Could you check a few things on this model? Use its own coordinates, in mm. A direction names the side the tool comes from. Round coordinates to 2 decimals unless told otherwise and drop trailing zeros. Write each loop counter-clockwise with the first axis right and the second up, starting at its lowest first coordinate (ties: lowest second). Pieces come first, ordered by that corner, then holes. Notation, with made-up numbers: (-12, 87.25) -> (14, 87.25) arc R16 ccw to (14, 94.25) -> close; hole circle Ø4 at (0.5, -15). An arc over 180 degrees is marked (long way). Answer in a Markdown table with one row per item.
from build123d import *

# Parameters (mm, degrees)
CUT_EXTRUDE1_START = -0.1
SKETCH2_R          = 7.95
SKETCH2_R_2        = 6.75
CUT_EXTRUDE1_DEPTH = 0.1


with BuildPart() as part:
    # Sketch1 → Revolve1 (revolve)
    with BuildSketch(Plane(origin=(0, 0, 0), x_dir=(0, 0, -1), z_dir=(1, 0, 0))):
        Polygon((0, 20), (9, 20), (9, 15.5), (8, 15.5), (8, 5), (6.75, 5), (6.75, 0), (0, 0), align=None)
    revolve(axis=Axis((0, 0, 0), (0, 1, 0)))

    # Sketch2 → Cut-Extrude1 (cut)
    with BuildSketch(Plane(origin=(0, 20, 0), x_dir=(1, 0, 0), z_dir=(0, 1, 0)).offset(CUT_EXTRUDE1_START)):
        with Locations(Location((0, 0, 0), (0, 0, 270))):
            Circle(SKETCH2_R)
        with Locations(Location((0, 0, 0), (0, 0, 90))):
            Circle(SKETCH2_R_2, mode=Mode.SUBTRACT)
    extrude(amount=CUT_EXTRUDE1_DEPTH, mode=Mode.SUBTRACT)


solid = part.part
1) Imagine slicing it at A-A, the plane x = 0. Please give me the cut outline in (y, z), plus the area to 3 significant figures.
Findings:
| item | result |
|---|---|
| outline | (0, -6.75) -> (5, -6.75) -> (5, -8) -> (15.5, -8) -> (15.5, -9) -> (20, -9) -> (20, -7.95) -> (19.9, -7.95) -> (19.9, -6.75) -> (20, -6.75) -> (20, 6.75) -> (19.9, 6.75) -> (19.9, 7.95) -> (20, 7.95) -> (20, 9) -> (15.5, 9) -> (15.5, 8) -> (5, 8) -> (5, 6.75) -> (0, 6.75) -> close |
| area | 316 mm^2 |
2) Imagine slicing it at C-C, the plane y = 16. Please give me the cut outline in (x, z).
Findings:
| item | result |
|---|---|
| outline | circle Ø18 at (0, 0) |
3) Thinking about a two-plate mould opening in X: for faces 1 (the face through (7.81, 10.18, 1.73)), 2 (the face through (-6, 19.9, -4)), 3 (the face through (6, 5, 4)), which applies, +X half, -X half, draft (parallel to the pull), parting line (faces both ways), or undercut?
Findings:
| item | result |
|---|---|
| face 1 | parting line |
| face 2 | undercut |
| face 3 | draft |
4) Imagine slicing it at B-B, the plane z = 0. Please give me the cut outline in (x, y), plus the area to 3 significant figures.
Findings:
| item | result |
|---|---|
| outline | (-9, 15.5) -> (-8, 15.5) -> (-8, 5) -> (-6.75, 5) -> (-6.75, 0) -> (6.75, 0) -> (6.75, 5) -> (8, 5) -> (8, 15.5) -> (9, 15.5) -> (9, 20) -> (7.95, 20) -> (7.95, 19.9) -> (6.75, 19.9) -> (6.75, 20) -> (-6.75, 20) -> (-6.75, 19.9) -> (-7.95, 19.9) -> (-7.95, 20) -> (-9, 20) -> close |
| area | 316 mm^2 |
5) For faces 4 (the face through (6.59, 2.46, 1.46)), 5 (the face through (0, 0, 0)), which set-ups out of +Z, -Z, +X, -X, +Y, -Y let a thin tool reach every point of the face, with its end or its side?
Findings:
| item | result |
|---|---|
| face 4 | -Y |
| face 5 | +Z, -Z, +X, -X, -Y |
6) Please list where these lines run through material, in increasing order: line 1 (X direction, y = 19.95, z = 0); line 2 (Y direction, x = -7.25, z = 4.5); line 3 (X direction, y = 12, z = 0).
Findings:
| item | result |
|---|---|
| line 1 | x = -9 to -7.95, -6.75 to 6.75, 7.95 to 9 |
| line 2 | y = 15.5 to 20 |
| line 3 | x = -8 to 8 |
7) For pin 1 (10 mm diameter, centred on y = 6.5, z = -1, fed in from +X); pin 2 (10 mm diameter, centred on y = 14.5, z = -6, fed in from +X); pin 3 (9 mm diameter, centred on x = -2, z = -0.5, fed in from -Y); pin 4 (3 mm diameter, centred on x = 0, y = 4, fed in from +Z), each with a flat end and sliding along its axis, tell me the tip position at first contact or that it passes through.
Findings:
| item | result |
|---|---|
| pin 1 | stops at x = 8 |
| pin 2 | stops at x = 8.93 |
| pin 3 | stops at y = 0 |
| pin 4 | stops at z = 8 |
